Part model, mm, in its own coordinate system. Face numbers are marked on the shaded views. A direction names the side the tool comes from. Round coordinates to 2 decimals unless told otherwise and drop trailing zeros. Write each loop counter-clockwise with the first axis right and the second up, starting at its lowest first coordinate (ties: lowest second). Pieces come first, ordered by that corner, then holes. Notation, with made-up numbers: (50.25, -34) -> (87.25, -34) arc R21 ccw to (87.25, -11) -> close; hole circle Ø4 at (-38, 7). An arc over 180 degrees is marked (long way). Return JSON: item names as keys, results as strings. Group by question number.
(1) Tool access for the marked faces 1 and 2: list every direction of +Z, -Z, +X, -X, +Y, -Y with a clear straight run to the whole face (end or side of a thin tool).
(2) Drill centre lines: L1, parallel to Y at x = 0, z = -13; L2, parallel to X at y = 15, z = 27.5; L3, parallel to Z at x = -2.5, y = 30.5. Where is each one in solid material? Low to high. Write a range as from..to.
(3) Drop flat-ended pins along their axis: pin 1 Ø10 at (x, y) = (16.5, 10.5) entering from -Z; pin 2 Ø12 at (x, z) = (-15.5, 16) entering from -Y; pin 3 Ø1.2 at (x, y) = (0, 0) entering from -Z; pin 4 Ø16.5 at (x, z) = (1.5, 25) entering from +Y. Give the stop position or say it passes through.
(4) Saw through at D-D (y = 0). List the corners of the cut face in (x, z).
(5) Saw through at A-A (x = 0). List the corners of the cut face in (y, z), plus the area to 3 significant figures.
(6) Saw through at C-C (z = 20.5). List the corners of the cut face in (x, y), plus the area to 3 significant figures.
(7) Saw through at B-B (y = -29). List the corners of the cut face in (x, z), plus the area to 3 significant figures.
(8) Mould opens along Y. For the marked faces 3, 4 and 5 say: +Y half, -Y half, draft (parallel to the pull), parting line (faces both ways), or undercut.
Autodesk Inventor part; units mm, degrees
ref_plane "YZ Plane" through (0, 0, 0) normal (1, 0, 0) x (0, 1, 0)
ref_plane "XZ Plane" through (0, 0, 0) normal (0, 1, 0) x (-1, 0, 0)
ref_plane "XY Plane" through (0, 0, 0) normal (0, 0, 1) x (1, 0, 0)
sketch "Sketch1" plane through (0, 0, 0) normal (0, 0, 1) x (1, 0, 0)
  circle A0 centre (0, 0) radius 58.5
  line L0 (0, 0) -> (0, 58.5) construction
  line L1 (0, 0) -> (-58.5, 0) construction
  line L2 (-21.9335, 54.2326) -> (-21.9335, -54.2326)
  line L3 (21.9335, 54.2326) -> (21.9335, -54.2326)
  point P0 (-54.2326, 21.9335)
  point P1 (54.2326, 21.9335)
  dimension "d0" = 117
  dimension "d53" = 21.9335
extrude "Extrusion1" add sketch "Sketch1" along normal blind 30 contours L3 A0 L2
sketch "Sketch2" plane through (0, 0, 0) normal (0, 0, -1) x (-1, 0, 0)
  circle A0 centre (0, 0) radius 6.5
  dimension "d4" = 13
extrude "Extrusion2" add sketch "Sketch2" along normal blind 15
sketch "Sketch6" plane through (0, 0, -15) normal (0, 0, -1) x (-1, 0, 0)
  circle A0 centre (0, 0) radius 1.15
  circle A1 centre (0, 0) radius 1.15
  line L0 (18.75, 0) -> (16.35, 0) construction
  line L1 (16.35, 0) -> (0, 0) construction
  line L2 (0, 0) -> (0, 3.75) construction
  circle A2 centre (0, 0) radius 3.9
  circle A3 centre (16.35, 0) radius 2.55
  line L3 (16.35, 2.55) -> (0.3241, 3.8865)
  line L4 (16.35, -2.55) -> (0.3241, -3.8865)
  point P0 (0, 3.75)
  dimension "d21" = 2.4
  dimension "d24" = 2.3
  dimension "d27" = 7.8
  dimension "d28" = 5.1
  dimension "d29" = 16.0259
  dimension "d30" = 16.0259
extrude "Extrusion5" [suppressed]
sketch "Sketch7" plane through (0, 0, -12.2) normal (0, 0, -1) x (-1, 0, 0)
  circle A0 centre (0, 0) radius 1.15
  dimension "d33" = 2.3
extrude "Extrusion6" [suppressed]
sketch "Sketch8" plane through (0, 0, 30) normal (0, 0, 1) x (1, 0, 0)
  line L0 (0, 0) -> (21.9335, 0) construction
  line L1 (0, 0) -> (15, 0)
  line L2 (15, 0) -> (15, 45)
  line L3 (15, 45) -> (-15, 45)
  line L4 (-15, 45) -> (-15, 0)
  line L5 (-15, 0) -> (0, 0)
  line L6 (-15, 0) -> (-15, -45)
  line L7 (-15, -45) -> (15, -45)
  line L8 (15, -45) -> (15, 0)
  dimension "d43" = 15
  dimension "d44" = 45
  dimension "d45" = 30
  dimension "d46" = 45
  dimension "d47" = 30
extrude "Extrusion7" cut sketch "Sketch8" against normal blind 15
sketch "Sketch9" plane through (0, 0, -15) normal (0, 0, -1) x (-1, 0, 0)
  circle A0 centre (0, 0) radius 3.5
  arc A1 (1.9, 14.1) -> (-1.8987, 14.0987) centre (0.0007, 14.05) ccw
  line L0 (0.0007, 15.95) -> (0.0007, 14.05)
  line L1 (0.0007, 14.05) -> (0, 0)
  circle A2 centre (0.0007, 14.05) radius 1.9
  line L2 (-1.8987, 14.0987) -> (-2.75, 2.1651)
  line L3 (-2.75, 2.1651) -> (-1.8987, 14.0987)
  line L4 (2.75, 2.1651) -> (1.9, 14.1)
  line L5 (2.75, 2.1651) -> (1.9, 14.1)
extrude "Extrusion8" cut sketch "Sketch9" against normal blind 3.8
sketch "Sketch10" plane through (0, 0, -11.2) normal (0, 0, -1) x (-1, 0, 0)
  circle A0 centre (0, 0) radius 1.15
  dimension "d50" = 2.3
extrude "Extrusion9" add sketch "Sketch10" along normal blind 3
properties part number "Sorting Gate Edited"
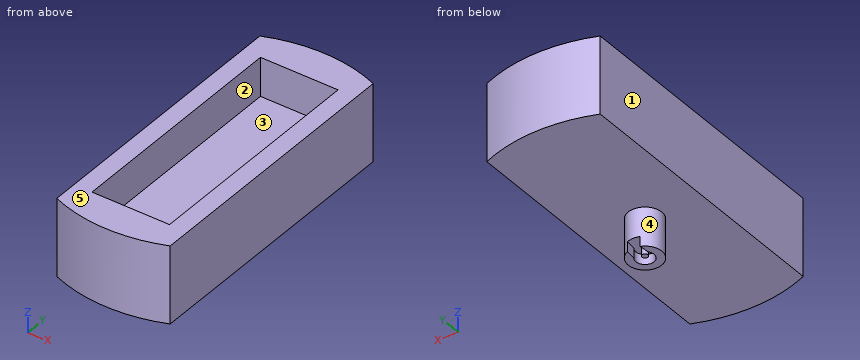
Computed values:
{
 "1": {"face 1": "+Z, -Z, -X, +Y, -Y", "face 2": "+Z"},
 "2": {"L1": "-6.5..-3.5, -1.15..1.15", "L2": "-21.93..-15, 15..21.93", "L3": "0..15"},
 "3": {"pin 1": "z = 0", "pin 2": "y = -57.72", "pin 3": "z = -14.2", "pin 4": "y = 58.5"},
 "4": {"outline": "(-21.93, 0) -> (-6.5, 0) -> (-6.5, -15) -> (-3.5, -15) -> (-3.5, -11.2) -> (-1.15, -11.2) -> (-1.15, -14.2) -> (1.15, -14.2) -> (1.15, -11.2) -> (3.5, -11.2) -> (3.5, -15) -> (6.5, -15) -> (6.5, 0) -> (21.93, 0) -> (21.93, 30) -> (15, 30) -> (15, 15) -> (-15, 15) -> (-15, 30) -> (-21.93, 30) -> close"},
 "5": {"outline": "(-58.5, 0) -> (-6.5, 0) -> (-6.5, -15) -> (-3.5, -15) -> (-3.5, -11.2) -> (-1.15, -11.2) -> (-1.15, -14.2) -> (1.15, -14.2) -> (1.15, -11.2) -> (6.5, -11.2) -> (6.5, 0) -> (58.5, 0) -> (58.5, 30) -> (45, 30) -> (45, 15) -> (-45, 15) -> (-45, 30) -> (-58.5, 30) -> close", "area": "2,320 mm2"},
 "6": {"outline": "(-21.93, -54.23) arc R58.5 ccw to (21.93, -54.23) -> (21.93, 54.23) arc R58.5 ccw to (-21.93, 54.23) -> close; hole (-15, -45) -> (15, -45) -> (15, 45) -> (-15, 45) -> close", "area": "2,310 mm2"},
 "7": {"outline": "(-21.93, 0) -> (21.93, 0) -> (21.93, 30) -> (15, 30) -> (15, 15) -> (-15, 15) -> (-15, 30) -> (-21.93, 30) -> close", "area": "866 mm2"},
 "8": {"face 3": "undercut", "face 4": "parting line", "face 5": "draft"}
}
